Geometry: final body of the model. Coordinates: model frame, mm. A direction names the side the tool comes from. Round coordinates to 2 decimals unless told otherwise and drop trailing zeros. Order: outer loops, then holes, each group sorted by start corner. A loop starts at its lowest first (then second) coordinate and runs counter-clockwise, first axis right, second up. Notation, with made-up numbers: (11.25, 81.25) - (52.25, 81.25) arc R31 cw to (52.25, 120.25) - close; hole circle Ø5 at (-5.5, 54). An arc over 180 degrees is marked (long way). Put each result on its own line as item: value. Start each with the question number.
(1) Section A-A (y = 2.5). Output: boundary loops of the cut face in (x, z), and give its area (3 significant figures).
(2) Material intervals for L1, parallel to Y at x = 4.75, z = -4.25; L2, parallel to Y at x = 1.5, z = -4.25; L3, parallel to Z at x = -0.5, y = 10.5, sorted ascending. Write a range as [from, to].
(3) Pull-direction query (Y, two-part tool) for faces 3 (the face through (4, 6.161, -2)), 4 (the face through (1, -1.339, 0)), 5 (the face through (4, 4.161, -3)), 6 (the face through (3.94, -0.85, -0.54)); classes: released by +Y, released by -Y, zero draft, split by the parting line, or undercut.
(4) Pin query (flat end, axial travel): P1, Ø1, axis at y = 5.5, z = -3, coming from the +X side; P2, Ø4, axis at x = -2.5, y = 5, coming from the +Z side; P3, Ø7.5, axis at x = 2, z = -0.5, coming from the +Y side; P4, Ø6, axis at x = -0.5, y = 2.5, coming from the +Z side. Return the tip coordinate at first contact, or that it passes through.
(5) Access query for faces 1 (the face through (2.65, 6.65, 2.77)), 2 (the face through (4.917, 2.14, -0.759)). Directions: +Z, -Z, +X, -X, +Y, -Y. A direction counts if a zero-diameter tool reaches every point of the face in a straight line with its end or side. Return the directions, or none.
from build123d import *


with BuildPart() as part:
    # Sketch1 → Revolve1 (revolve)
    with BuildSketch(Plane.XY, mode=Mode.PRIVATE) as revolve1_sk:
        with BuildLine():
            Line((-6.282911506, 19.040573868), (-1.5, 7.161021792))
            Line((-1.5, 7.161021792), (-1.5, 6.161021792))
            Line((-1.5, 6.161021792), (-2, 6.161021792))
            Line((-2, 6.161021792), (-2, 4.161021792))
            Line((-2, 4.161021792), (-5, 4.161021792))
            Line((-5, 4.161021792), (-5, 3.661021792))
            Line((-5, 3.661021792), (-2, 3.661021792))
            Line((-2, 3.661021792), (-2, 0.661021792))
            Line((-2, 0.661021792), (-1, -0.338978208))
            Line((-1, -0.338978208), (-1, -1.338978208))
            Line((-1, -1.338978208), (1.5, -1.338978208))
            Line((1.5, -1.338978208), (1.5, 23.340167272))
            ThreePointArc((1.5, 23.340167272), (-1.004003623, 23.36233677), (-3.5, 23.161021792))
            ThreePointArc((-3.5, 23.161021792), (-5.986095711, 21.840107292), (-6.282911506, 19.040573868))
        make_face()
    revolve(revolve1_sk.sketch.rotate(Axis((1.5, 32.403614304, 0), (0, -1, 0)), 270), axis=Axis((1.5, 32.403614304, 0), (0, -1, 0)))


solid = part.part
Checks:
1. outline: circle Ø7 at (1.5, 0)
1. area: 38.5 mm²
2. L1: y = [3.66, 4.16], [13, 23.14]
2. L2: y = [3.66, 4.16], [10.27, 23.25]
2. L3: z = [-3.86, 3.86]
3. face 3: undercut
3. face 4: released by -Y
3. face 5: undercut
3. face 6: zero draft
4. P1: stops at x = 3.95
4. P2: stops at z = 6.12
4. P3: stops at y = 23.38
4. P4: stops at z = 6.5
5. face 1: none
5. face 2: -Y
